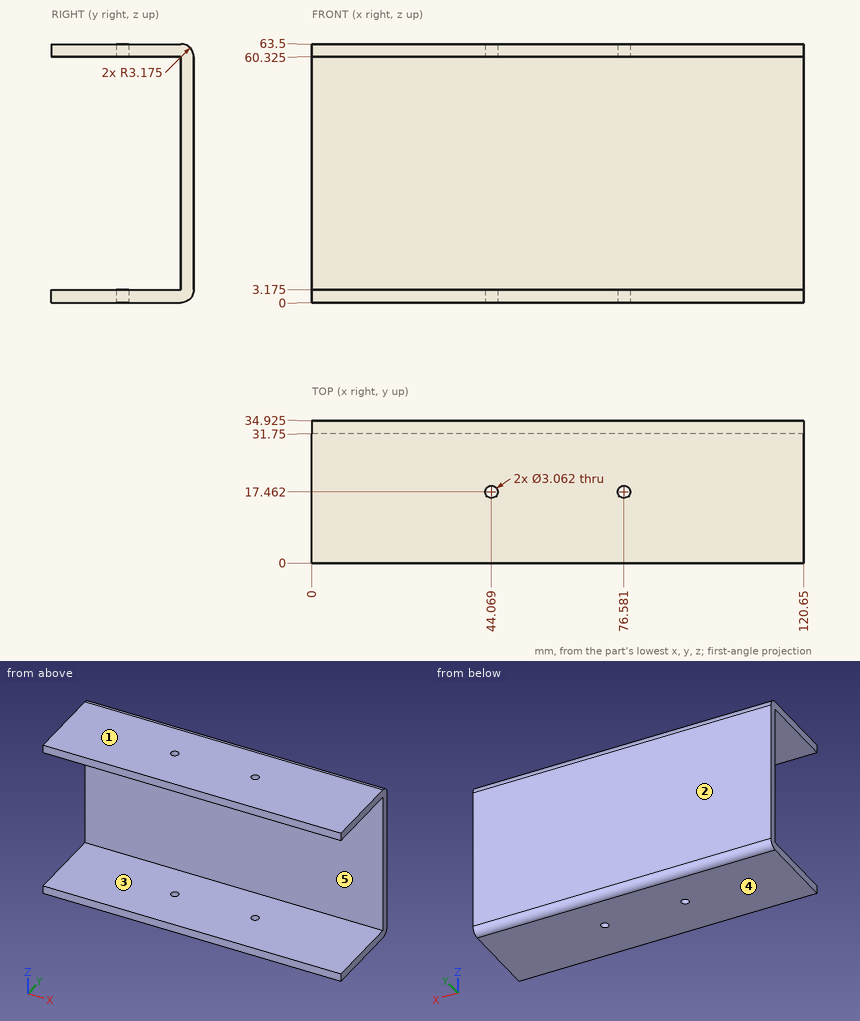
The figure shows three views and two pictorial views of one solid part (mm, origin at its lowest corner). Answer the questions. A direction names the side the tool comes from. Give positions to 0.01 mm unless a question says otherwise; leave off trailing zeros.
Q1. Given pin 1 (3 mm diameter, centred on x = 36, y = 9, fed in from -Z); pin 2 (10 mm diameter, centred on x = 44, z = 38, fed in from -Y), each flat-ended and moving along its own axis, determine where each tip first touches the part or whether it passes through.
Answer:
pin 1: stops at z = 0
pin 2: stops at y = 31.75
Q2. A tool of negligible diameter and unlimited length cuts with its end or side. For the marked faces 4 and 5, from which of +Z, -Z, +X, -X, +Y, -Y can it reach the whole face along a straight path? Write none if from no direction.
Answer:
face 4: -Z, +X, -X, +Y, -Y
face 5: +X, -X, -Y
Q3. A straight line is drawn through the part: L1, parallel to Z at x = 87.5, y = 8.5 (1 decimal). Find the intervals that lie inside material, in ascending order.
Answer:
L1: z = 0 to 3.2, 60.3 to 63.5
Q4. For a pull along Z with two mould halves and no side action, classify the marked faces 1, 2 and 3 as released by +Z, released by -Z, zero draft, split by the parting line, or undercut.
Answer:
face 1: released by +Z
face 2: zero draft
face 3: undercut
